```python
from build123d import *

# Parameters (mm, degrees)
SKETCH1_W           = 12.3698
SKETCH1_H           = 20.066
BOSS_EXTRUDE1_DEPTH = 2.5908
SKETCH2_R           = 1.6256
BOSS_EXTRUDE2_DEPTH = 3.175
CHAMFER1_SIZE       = 0.127


with BuildPart() as part:
    # Sketch1 → Boss-Extrude1 (new body)
    with BuildSketch(Plane(origin=(0, 0, 0), x_dir=(1, 0, 0), z_dir=(0, 1, 0))):
        Rectangle(SKETCH1_W, SKETCH1_H)
    extrude(amount=BOSS_EXTRUDE1_DEPTH)

    # Sketch2 → Boss-Extrude2 (add)
    with BuildSketch(Plane(origin=(0, 2.5908, 0), x_dir=(1, 0, 0), z_dir=(0, 1, 0))):
        with Locations(Location((3.3909, 7.55015, 0), (0, 0, 270))):
            Circle(SKETCH2_R)
        with Locations(Location((3.3909, -7.55015, 0), (0, 0, 90))):
            Circle(SKETCH2_R)
    extrude(amount=BOSS_EXTRUDE2_DEPTH)

    # Chamfer1
    chamfer1_edges = [part.edges().sort_by_distance(p)[0] for p in [
        (3.3909, 5.7658, -9.17575),
        (3.3909, 5.7658, 9.17575),
    ]]
    chamfer(chamfer1_edges, length=CHAMFER1_SIZE)


solid = part.part
```
The listing builds one solid part. Answer for the finished solid, in the listing's coordinates (mm). A direction names the side the tool comes from. Coordinates: 2 decimals unless noted, no trailing zeros. Write each loop counter-clockwise with the first axis right and the second up, starting at its lowest first coordinate (ties: lowest second). Pieces come first, ordered by that corner, then holes. Notation, with made-up numbers: (-27.5, -7) - (31.5, -7) arc R19 cw to (31.5, 9) - close; hole circle Ø8 at (2, 25). An arc over 180 degrees is marked (long way). Return JSON: item names as keys, results as strings. Group by question number.
Q1. The part is cut by section A-A on y = 3.3. Write down the section's boundary in (x, z).
Q2. Find the intervals of material crossed by line 1 along Y through (x, z) = (-2, -4.75), in increasing order. Write a range as [from, to].
Q3. The part is cut by section B-B on x = -2. Write down the section's boundary in (y, z).
Q4. The part is cut by section C-C on z = -2.5. Write down the section's boundary in (x, y).
Q5. Which of the six approach directions +Z, -Z, +X, -X, +Y, -Y give full straight-line access (tool end or side, diameter ignored) to faces 4 (the flat face through (3, 5.766, 8)), 5 (the cylindrical face through (2.768, 4.093, -6.049))?
Q6. Flat-ended cylindrical pins translate along their axes: pin 1 Ø1 at (y, z) = (5, -2) entering from +X; pin 2 Ø3 at (y, z) = (4.5, -7) entering from -X. Find the tip coordinate at first contact, or state that the pin passes through.
Q7. For a pull along Z with two mould halves and no side action, classify faces 1 (the flat face through (0, 0, 0)), 2 (the cylindrical face through (4.833, 4.093, 6.8)), 3 (the flat face through (0, 1, -10.033)) as +Z half, -Z half, draft (parallel to the pull), parting line (faces both ways), or undercut.
Evaluation:
{
 "1": {"outline": "circle Ø3.25 at (3.39, -7.55); circle Ø3.25 at (3.39, 7.55)"},
 "2": {"line 1": "y = [0, 2.59]"},
 "3": {"outline": "(0, -10.03) - (2.59, -10.03) - (2.59, 10.03) - (0, 10.03) - close"},
 "4": {"outline": "(-6.18, 0) - (6.18, 0) - (6.18, 2.59) - (-6.18, 2.59) - close"},
 "5": {"face 4": "+Z, -Z, +X, -X, +Y", "face 5": "+Y"},
 "6": {"pin 1": "passes through", "pin 2": "stops at x = 1.77"},
 "7": {"face 1": "draft", "face 2": "undercut", "face 3": "-Z half"}
}
